Geometry check sheet. Reference: the model listing, model coordinates, mm. A direction names the side the tool comes from. Coordinates: 2 decimals unless noted, no trailing zeros. Write each loop counter-clockwise with the first axis right and the second up, starting at its lowest first coordinate (ties: lowest second). Pieces come first, ordered by that corner, then holes. Notation, with made-up numbers: (62, 57.5) -> (97, 57.5) arc R30 ccw to (97, 79.5) -> close; hole circle Ø11 at (36, 66.5). An arc over 180 degrees is marked (long way). Use a Markdown table: item, result.
```python
from build123d import *

# Parameters (mm, degrees)
SKETCH1_R               = 1
SKETCH1_R_2             = 1.5
BOSS_EXTRUDE1_DEPTH     = 8
SKETCH2_R               = 1.5
CUT_EXTRUDE1_DEPTH      = 20.25
BOSS_EXTRUDE2_DEPTH     = 14.75
SKETCH5_R               = 3.075
CUT_EXTRUDE2_DEPTH      = 5.5
CUT_EXTRUDE2_DEPTH_BACK = 2
CHAMFER2_SIZE           = 2
FILLET1_R               = 10
SKETCH6_R               = 1.225
CUT_EXTRUDE3_DEPTH      = 5


with BuildPart() as part:
    # Sketch1 → Boss-Extrude1 (new body)
    with BuildSketch(Plane.XY):
        with BuildLine():
            Line((34.6, 7.35), (34.6, 0))
            Line((34.6, 0), (39.45, 0))
            Line((39.45, 0), (39.45, 14.75))
            Line((39.45, 14.75), (14.598076211, 14.75))
            ThreePointArc((14.598076211, 14.75), (12, 19.25), (9.401923789, 14.75))
            Line((9.401923789, 14.75), (-9.401923789, 14.75))
            ThreePointArc((-9.401923789, 14.75), (-12, 19.25), (-14.598076211, 14.75))
            Line((-14.598076211, 14.75), (-39.45, 14.75))
            Line((-39.45, 14.75), (-39.45, 0))
            Line((-39.45, 0), (-34.6, 0))
            Line((-34.6, 0), (-34.6, 7.35))
            Line((-34.6, 7.35), (34.6, 7.35))
        make_face()
        with Locations((-5, 11.75)):
            Circle(SKETCH1_R, mode=Mode.SUBTRACT)
        with Locations((5, 11.75)):
            Circle(SKETCH1_R, mode=Mode.SUBTRACT)
        with Locations((27, 11.75)):
            Circle(SKETCH1_R, mode=Mode.SUBTRACT)
        with Locations((-27, 11.75)):
            Circle(SKETCH1_R, mode=Mode.SUBTRACT)
        with Locations((12, 16.25)):
            Circle(SKETCH1_R_2, mode=Mode.SUBTRACT)
        with Locations((-12, 16.25)):
            Circle(SKETCH1_R_2, mode=Mode.SUBTRACT)
    extrude(amount=BOSS_EXTRUDE1_DEPTH)

    # Sketch2 → Cut-Extrude1 (cut, through all)
    with BuildSketch(Plane.XZ):
        with Locations((-37, 4)):
            Circle(SKETCH2_R)
        with Locations((37, 4)):
            Circle(SKETCH2_R)
    extrude(amount=-CUT_EXTRUDE1_DEPTH, mode=Mode.SUBTRACT)

    # Sketch3 → Boss-Extrude2 (add)
    with BuildSketch(Plane(origin=(0, 14.75, 0), x_dir=(1, 0, 0), z_dir=(0, 1, 0))):
        with BuildLine():
            Line((39.45, -8), (39.45, 0))
            ThreePointArc((39.45, 0), (41.690682253, -4), (39.45, -8))
        make_face()
        with BuildLine():
            Line((-39.45, -8), (-39.45, 0))
            ThreePointArc((-39.45, 0), (-41.690682253, -4), (-39.45, -8))
        make_face()
    extrude(amount=-BOSS_EXTRUDE2_DEPTH)

    # Sketch5 → Cut-Extrude2 (cut, two sides)
    with BuildSketch(Plane(origin=(0, 14.75, 0), x_dir=(1, 0, 0), z_dir=(0, 1, 0))) as cut_extrude2_sk:
        with Locations((37, -4)):
            Circle(SKETCH5_R)
        with Locations((-37, -4)):
            Circle(SKETCH5_R)
    extrude(amount=CUT_EXTRUDE2_DEPTH, mode=Mode.SUBTRACT)
    extrude(cut_extrude2_sk.sketch, amount=-CUT_EXTRUDE2_DEPTH_BACK, mode=Mode.SUBTRACT)

    # Chamfer2
    chamfer2_edges = [part.edges().sort_by_distance(p)[0] for p in [
        (-34.6, 7.35, 4),
        (34.6, 7.35, 4),
    ]]
    chamfer(chamfer2_edges, length=CHAMFER2_SIZE)

    # Fillet1
    fillet1_edges = [part.edges().sort_by_distance(p)[0] for p in [
        (-14.598076211, 14.75, 4),
        (-9.401923789, 14.75, 4),
        (9.401923789, 14.75, 4),
        (14.598076211, 14.75, 4),
    ]]
    fillet(fillet1_edges, radius=FILLET1_R)

    # Sketch6 → Cut-Extrude3 (cut)
    with BuildSketch(Plane.XY.offset(8)):
        with Locations((-27, 11.75)):
            Circle(SKETCH6_R)
        with Locations((-5, 11.75)):
            Circle(SKETCH6_R)
        with Locations((5, 11.75)):
            Circle(SKETCH6_R)
        with Locations((27, 11.75)):
            Circle(SKETCH6_R)
    extrude(amount=-CUT_EXTRUDE3_DEPTH, mode=Mode.SUBTRACT)


solid = part.part
```
Item 1: Depth check by flat-ended pin: P1, Ø1.8, axis at x = -37, z = 4, coming from the -Y side; P2, Ø1.5, axis at x = -22.5, z = 4.5, coming from the -Y side; P3, Ø3, axis at x = -5, y = 11.75, coming from the +Z side; P4, Ø1.3, axis at x = 1, z = 3.5, coming from the +Y side. Enter the tip coordinate at first touch or a pass-through.
Answer block:
| item | result |
|---|---|
| P1 | passes through |
| P2 | stops at y = 7.35 |
| P3 | stops at z = 8 |
| P4 | stops at y = 14.75 |
Item 2: Section check D-D on x = 27. Record the boundary of the cut face in (y, z) (3 decimals).
Answer block:
| item | result |
|---|---|
| outline | (7.35, 0) -> (10.75, 0) -> (10.75, 3) -> (10.525, 3) -> (10.525, 8) -> (7.35, 8) -> close; (12.75, 0) -> (14.75, 0) -> (14.75, 8) -> (12.975, 8) -> (12.975, 3) -> (12.75, 3) -> close |
Item 3: Tool access check on faces 4 (the cylindrical face through (-6.27, 15.63, 4.06)), 5 (the flat face through (30, 14.75, 4)), 6 (the cylindrical face through (28.168, 12.118, 5.535)), 7 (the flat face through (-33.61, 6.34, 3.94)). Record the directions out of +Z, -Z, +X, -X, +Y, -Y that give a thin tool (end or side, any length) a straight path to the whole face; none if there is none.
Answer block:
| item | result |
|---|---|
| face 4 | +Z, -Z, +Y |
| face 5 | +Z, -Z, +X, +Y |
| face 6 | +Z |
| face 7 | +Z, -Z, -Y |
Item 4: Section check B-B on z = 4. Count the separate pieces of the cut face and the enclosed holes in it, then the cut area to 3 significant figures.
Answer block:
| item | result |
|---|---|
| separate pieces | 3 |
| enclosed holes | 6 |
| area | 661 mm^2 |
Item 5: Section check C-C on y = 8.75. Record the boundary of the cut face in (x, z).
Answer block:
| item | result |
|---|---|
| outline | (-39.45, 0) -> (39.45, 0) arc R4.69 ccw to (39.45, 8) -> (-39.45, 8) arc R4.69 ccw to start; hole circle Ø3 at (-37, 4); hole circle Ø3 at (37, 4) |
Item 6: Thickness scan on L1, parallel to X at y = 13.95, z = 4 (3 decimals); L2, parallel to Z at x = -37, y = 11; L3, parallel to Y at x = -27, z = 1.85. Record the ranges inside material, lowest first. Write a range as [from, to].
Answer block:
| item | result |
|---|---|
| L1 | x = [-41.691, -40.075], [-33.925, 33.925], [40.075, 41.691] |
| L2 | z = [0, 2.5], [5.5, 8] |
| L3 | y = [7.35, 10.75], [12.75, 14.75] |
Item 7: Section check A-A on x = 37. Record the boundary of the cut face in (y, z) (3 decimals), then the cut area to 4 significant figures.
Answer block:
| item | result |
|---|---|
| outline | (0, 0) -> (14.75, 0) -> (14.75, 0.925) -> (12.75, 0.925) -> (12.75, 2.5) -> (0, 2.5) -> close; (0, 5.5) -> (12.75, 5.5) -> (12.75, 7.075) -> (14.75, 7.075) -> (14.75, 8) -> (0, 8) -> close |
| area | 67.45 mm^2 |
Item 8: Mould release check, pull along Z, two halves, no side actions. Record for faces 1 (the cylindrical face through (-6.224, 11.804, 5.535)), 2 (the flat face through (-1, 10, 8)), 3 (the cylindrical face through (39.84, 13.76, 5.18)): +Z half, -Z half, draft (parallel to the pull), parting line (faces both ways), or undercut.
Answer block:
| item | result |
|---|---|
| face 1 | draft |
| face 2 | +Z half |
| face 3 | undercut |
